Part model, mm, in its own coordinate system. Give positions to 0.01 mm unless a question says otherwise; leave off trailing zeros. Write each loop counter-clockwise with the first axis right and the second up, starting at its lowest first coordinate (ties: lowest second). Pieces come first, ordered by that corner, then holes. Notation, with made-up numbers: M 26.25,-9.5 L 72.25,-9.5 A33 ccw 72.25,18.5 Z; hole C 1.25,7 d10. An arc over 180 degrees is marked long. Use a Markdown table: item, result.
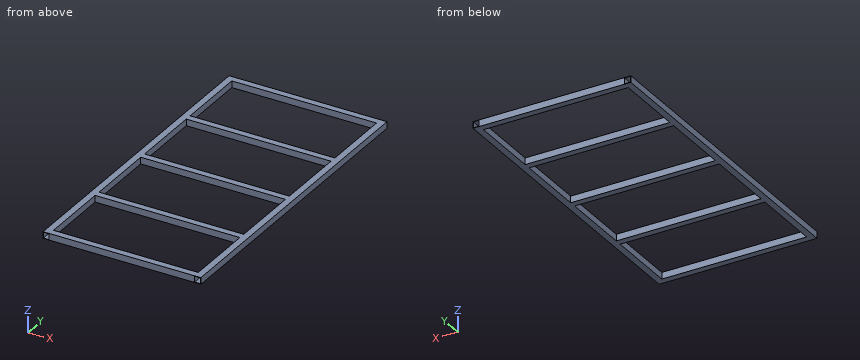
```python
from build123d import *

# Parameters (mm, degrees)
F0_W     = 44.704
F0_H     = 44.704
F0_W_2   = 50.8
F0_H_2   = 50.8
F1_DEPTH = 2438.4
F2_DEPTH = 2438.4
F3_W     = 50.8
F3_H     = 50.8
F3_W_2   = 44.704
F3_H_2   = 44.704
F4_DEPTH = 1117.6


with BuildPart() as f1:
    # F0 (on Front) → F1 (new body)
    with BuildSketch(Plane.XZ):
        with Locations((-584.2, 25.4)):
            Rectangle(F0_W, F0_H)
        with Locations((-584.2, 25.4)):
            Rectangle(F0_W_2, F0_H_2)
        with Locations((-584.2, 25.4)):
            Rectangle(F0_W, F0_H, mode=Mode.SUBTRACT)
        with Locations((584.2, 25.4)):
            Rectangle(F0_W, F0_H)
        with Locations((584.2, 25.4)):
            Rectangle(F0_W_2, F0_H_2)
        with Locations((584.2, 25.4)):
            Rectangle(F0_W, F0_H, mode=Mode.SUBTRACT)
    extrude(amount=F1_DEPTH)

    # F0 (on Front) → F2 (cut)
    with BuildSketch(Plane.XZ):
        with Locations((-584.2, 25.4)):
            Rectangle(F0_W, F0_H)
        with Locations((584.2, 25.4)):
            Rectangle(F0_W, F0_H)
    extrude(amount=F2_DEPTH, mode=Mode.SUBTRACT)

    # F3 (on face) → F4 (join, through all)
    with BuildSketch(Plane.YZ.offset(-558.8)):
        with Locations((-2413, 25.4)):
            Rectangle(F3_W, F3_H)
        with Locations((-2413, 25.4)):
            Rectangle(F3_W_2, F3_H_2, mode=Mode.SUBTRACT)
        with Locations((-1816.1, 25.4)):
            Rectangle(F3_W, F3_H)
        with Locations((-1816.1, 25.4)):
            Rectangle(F3_W_2, F3_H_2, mode=Mode.SUBTRACT)
        with Locations((-1219.2, 25.4)):
            Rectangle(F3_W, F3_H)
        with Locations((-1219.2, 25.4)):
            Rectangle(F3_W_2, F3_H_2, mode=Mode.SUBTRACT)
        with Locations((-622.3, 25.4)):
            Rectangle(F3_W, F3_H)
        with Locations((-622.3, 25.4)):
            Rectangle(F3_W_2, F3_H_2, mode=Mode.SUBTRACT)
        with Locations((-25.4, 25.4)):
            Rectangle(F3_W, F3_H)
        with Locations((-25.4, 25.4)):
            Rectangle(F3_W_2, F3_H_2, mode=Mode.SUBTRACT)
    extrude(amount=F4_DEPTH)


solid = f1.part
```
1. Drill centre lines: L1, parallel to X at y = -1235, z = 27; L2, parallel to Y at x = 151, z = 48; L3, parallel to Z at x = 260.5, y = -1800. Where is each one in solid material? Low to high.
Findings below:
| item | result |
|---|---|
| L1 | -609.6 to -606.55, -561.85 to -558.8, 558.8 to 561.85, 606.55 to 609.6 |
| L2 | -2438.4 to -2387.6, -1841.5 to -1790.7, -1244.6 to -1193.8, -647.7 to -596.9, -50.8 to 0 |
| L3 | 0 to 3.05, 47.75 to 50.8 |
2. Cut at B-B, the plane x = 52. State how many separate pieces and enclosed holes the cut face has, then the cut area to 3 significant figures.
Findings below:
| item | result |
|---|---|
| separate pieces | 5 |
| enclosed holes | 5 |
| area | 2,910 mm2 |
3. Cut at A-A, the plane y = -1276.5. Give the cut face in (x, z), then the cut area to 3 significant figures.
Findings below:
| item | result |
|---|---|
| outline | M -609.6,0 L -558.8,0 L -558.8,50.8 L -609.6,50.8 Z; M 558.8,0 L 609.6,0 L 609.6,50.8 L 558.8,50.8 Z; hole M -606.55,3.05 L -561.85,3.05 L -561.85,47.75 L -606.55,47.75 Z; hole M 561.85,3.05 L 606.55,3.05 L 606.55,47.75 L 561.85,47.75 Z |
| area | 1,160 mm2 |
